Print and shaded views of the part. All mm, measured from the part's lowest x, y and z. Round coordinates to 2 decimals unless told otherwise and drop trailing zeros. Order: outer loops, then holes, each group sorted by start corner. A loop starts at its lowest first (then second) coordinate and runs counter-clockwise, first axis right, second up.
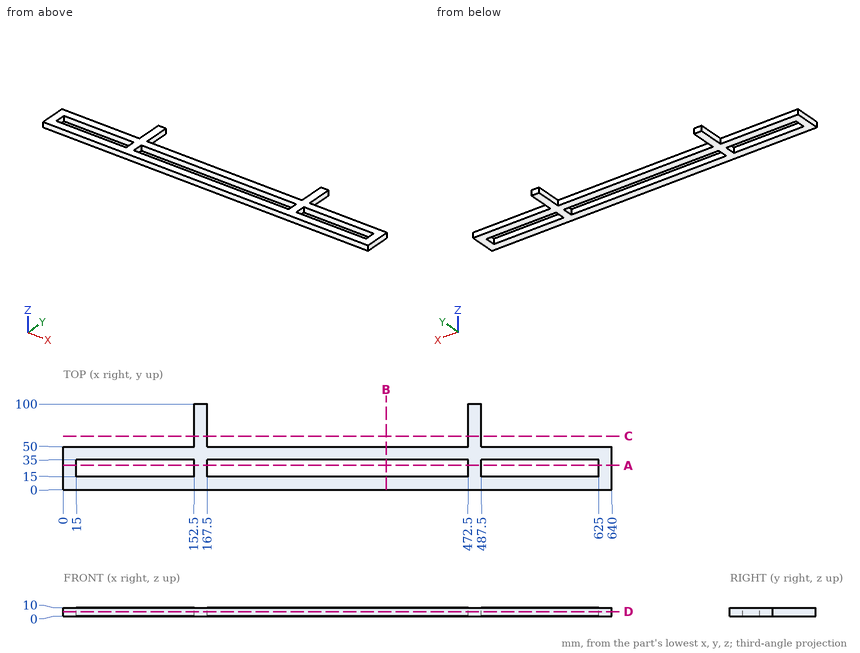
1. Cut at B-B, the plane x = 376.5. Write the cut outline in (y, z).
2. Cut at D-D, the plane z = 5.5. Write the cut outline in (x, y), and give its area (3 significant figures).
3. Cut at A-A, the plane y = 28.5. Write the cut outline in (x, z), and give its area (3 significant figures).
4. Drill centre lines: line 1 (X direction, y = 24.5, z = 3.25); line 2 (Y direction, x = 490, z = 8.75); line 3 (X direction, y = 91, z = 6.75). Where is each one in solid material? Low to high.
5. Pin check, flat tips, straight feed: P1, Ø4, axis at y = 83.5, z = 4.5, coming from the -X side; P2, Ø3, axis at x = 587.5, z = 2.5, coming from the +Y side; P3, Ø5, axis at y = 72.5, z = 5.5, coming from the +X side. Stop position of each tip, or through.
6. Cut at C-C, the plane y = 62.5. Write the cut outline in (x, z).
Outcome:
1. outline: (0, 0) - (15, 0) - (15, 10) - (0, 10) - close; (35, 0) - (50, 0) - (50, 10) - (35, 10) - close
2. outline: (0, 0) - (640, 0) - (640, 50) - (487.5, 50) - (487.5, 100) - (472.5, 100) - (472.5, 50) - (167.5, 50) - (167.5, 100) - (152.5, 100) - (152.5, 50) - (0, 50) - close; hole (15, 15) - (152.5, 15) - (152.5, 35) - (15, 35) - close; hole (167.5, 15) - (472.5, 15) - (472.5, 35) - (167.5, 35) - close; hole (487.5, 15) - (625, 15) - (625, 35) - (487.5, 35) - close
2. area: 21,900 mm2
3. outline: (0, 0) - (15, 0) - (15, 10) - (0, 10) - close; (152.5, 0) - (167.5, 0) - (167.5, 10) - (152.5, 10) - close; (472.5, 0) - (487.5, 0) - (487.5, 10) - (472.5, 10) - close; (625, 0) - (640, 0) - (640, 10) - (625, 10) - close
3. area: 600 mm2
4. line 1: x = 0 to 15, 152.5 to 167.5, 472.5 to 487.5, 625 to 640
4. line 2: y = 0 to 15, 35 to 50
4. line 3: x = 152.5 to 167.5, 472.5 to 487.5
5. P1: stops at x = 152.5
5. P2: stops at y = 50
5. P3: stops at x = 487.5
6. outline: (152.5, 0) - (167.5, 0) - (167.5, 10) - (152.5, 10) - close; (472.5, 0) - (487.5, 0) - (487.5, 10) - (472.5, 10) - close
